from build123d import *

# Parameters (mm, degrees)
PAD_DEPTH = 180


with BuildPart() as pad:
    # Sketch → Pad (new body)
    with BuildSketch(Plane.XY):
        with BuildLine():
            Line((-4.01, 0), (-12.01, 0))
            Line((-12.01, 0), (-12.01, -6.353146))
            Line((-12.01, -6.353146), (-17, -11.343146))
            Line((-17, -11.343146), (-20, -11.343146))
            Line((-20, -11.343146), (-20, -5))
            Line((-20, -5), (-25, -5))
            Line((-25, -5), (-25, -22))
            ThreePointArc((-25, -22), (-24.12132, -24.12132), (-22, -25))
            Line((-22, -25), (-5, -25))
            Line((-5, -25), (-5, -20))
            Line((-5, -20), (-11.343146, -20))
            Line((-11.343146, -20), (-11.343146, -17))
            Line((-11.343146, -17), (-6.353146, -12.01))
            Line((-6.353146, -12.01), (0, -12.01))
            Line((0, -12.01), (0, -4.01))
            ThreePointArc((-4.01, 0), (-2.835498, -2.835498), (0, -4.01))
        make_face()
    extrude(amount=PAD_DEPTH)


with BuildPart() as part_mirroring:
    # Part__Mirroring: instance of Pad
    add(pad.part.mirror(Plane(origin=(0, 0, 0), x_dir=(1, 0, 0), z_dir=(0, 1, 0))))


with BuildPart() as fusion:
    # Fusion base: copy of Pad
    add(pad.part)

    # Fusion: union Part__Mirroring
    add(part_mirroring.part)


with BuildPart() as obj1:
    # Part__Mirroring001: instance of Fusion
    add(fusion.part.mirror(Plane(origin=(0, 0, 0), x_dir=(0, -1, 0), z_dir=(1, 0, 0))))

    # Fusion001: union Fusion
    add(fusion.part)


solid = obj1.part
The listing builds one solid part. Answer for the finished solid, in the listing's coordinates (mm). A direction names the side the tool comes from. Round coordinates to 2 decimals unless told otherwise and drop trailing zeros. Order: outer loops, then holes, each group sorted by start corner. A loop starts at its lowest first (then second) coordinate and runs counter-clockwise, first axis right, second up. Notation, with made-up numbers: (25.25, 80.5) - (76.25, 80.5) arc R15 cw to (76.25, 90.5) - close; hole circle Ø5 at (-20, -33). An arc over 180 degrees is marked (long way). Write item = value, one per line. Start each with the question number.
1) For a pull along Y with two mould halves and no side action, classify faces 5 (the cylindrical face through (-24.14, -24.1, 88.74)), 6 (the flat face through (5, 0, 0)), 7 (the flat face through (11.343, 19, 89)) as released by +Y, released by -Y, zero draft, split by the parting line, or undercut.
2) For faces 1 (the cylindrical face through (24.14, -24.1, 88.74)), 2 (the flat face through (22, 5, 89)), 3 (the flat face through (-22, 5, 89)), 4 (the flat face through (8, 20, 89)), determine the directions among +Z, -Z, +X, -X, +Y, -Y from which every point of the face is accessible in a straight line to the end or side of a thin tool.
3) Straight lines are drawn through the part: L1, parallel to X at y = -8.5, z = 11; L2, parallel to Y at x = -9.5, z = 97; L3, parallel to Y at x = 18.5, z = 95.5. For each, find the intervals that lie inside material, in ascending order.
4) Section A-A, the plane y = 9.5 is taken. Write down the section's boundary in (x, z), plus the area to 3 significant figures.
5) Given pin 1 (6.5 mm diameter, centred on y = -0.5, z = 71.5, fed in from -X); pin 2 (4 mm diameter, centred on x = -2.5, z = 48, fed in from +Y); pin 3 (1.5 mm diameter, centred on y = -23, z = 95.5, fed in from +X), each flat-ended and moving along its own axis, determine where each tip first touches the part or whether it passes through.
Results list:
q1.face_5 = released by -Y
q1.face_6 = zero draft
q1.face_7 = undercut
q2.face_1 = +Z, -Z, +X, -Y
q2.face_2 = +Z, -Z, +X
q2.face_3 = +Z, -Z, -X
q2.face_4 = +Z, -Z
q3.L1 = -25 to -20, -14.16 to 14.16, 20 to 25
q3.L2 = -25 to -20, -15.16 to 15.16, 20 to 25
q3.L3 = -25 to -11.34, 11.34 to 25
q4.outline = (-25, 0) - (-20, 0) - (-20, 180) - (-25, 180) - close; (-15.16, 0) - (15.16, 0) - (15.16, 180) - (-15.16, 180) - close; (20, 0) - (25, 0) - (25, 180) - (20, 180) - close
q4.area = 7,260 mm^2
q5.pin_1 = -12.01
q5.pin_2 = 12.01
q5.pin_3 = 24.99
